```python
from build123d import *

# Parameters (mm, degrees)
F0_W          = 128.129378
F0_H          = 77.922702
F1_DEPTH      = 254
F1_DEPTH_BACK = 25.4
F2_W          = 85.559396
F2_H          = 132.324406
F3_DEPTH      = 254
F4_W          = 107.157492
F4_H          = 126.91684
F5_DEPTH      = 127


with BuildPart() as f1:
    # F0 (on Top) → F1 (new body, two sides)
    with BuildSketch(Plane.XY) as f1_sk:
        Rectangle(F0_W, F0_H)
    extrude(amount=F1_DEPTH)
    extrude(f1_sk.sketch, amount=-F1_DEPTH_BACK)

    # F2 (on Front) → F3 (cut)
    with BuildSketch(Plane.XZ):
        Rectangle(F2_W, F2_H)
    extrude(amount=F3_DEPTH, mode=Mode.SUBTRACT)

    # F4 (on Front) → F5 (cut, symmetric)
    with BuildSketch(Plane.XZ):
        with Locations((0, 155.446574)):
            Rectangle(F4_W, F4_H)
    extrude(amount=F5_DEPTH, both=True, mode=Mode.SUBTRACT)


solid = f1.part
```
Geometry check sheet. Reference: the model listing, model coordinates, mm. A direction names the side the tool comes from. Round coordinates to 2 decimals unless told otherwise and drop trailing zeros. Order: outer loops, then holes, each group sorted by start corner. A loop starts at its lowest first (then second) coordinate and runs counter-clockwise, first axis right, second up. Notation, with made-up numbers: M -14.5,-39 L 15.5,-39 A19 cw 15.5,-11 Z; hole C 7.5,31.25 d3. An arc over 180 degrees is marked long. Answer as CSV lines item,"result".
1) Gauge pin test, flat end, axial feed: pin 1 Ø1.5 at (x, y) = (34.5, -11) entering from -Z. Record the tip position at first contact, or that the pin passes through.
Entries:
pin 1,"z = 66.16"
2) Mould release check, pull along X, two halves, no side actions. Record for faces 1 (the face through (64.065, -1, 116)), 2 (the face through (-64.065, -1, 116)), 3 (the face through (-1, 0, 21)), 4 (the face through (-1, 1, 254)): +X half, -X half, draft (parallel to the pull), parting line (faces both ways), or undercut.
Entries:
face 1,"+X half"
face 2,"-X half"
face 3,"undercut"
face 4,"draft"
3) Thickness scan on probe 1 along X at (y, z) = (-9, 188.5); probe 2 along X at (y, z) = (-16, 41); probe 3 along Z at (x, y) = (-25, -5.5) (3 decimals). Record the ranges inside material, lowest first. Write a range as [from, to].
Entries:
probe 1,"[-64.06, -53.58], [53.58, 64.06]"
probe 2,"[-64.06, -42.78], [42.78, 64.06]"
probe 3,"[66.162, 91.988], [218.905, 254]"
4) Sectioned sample at A-A on z = 155. Record the cut outline in (x, y), and give its area (3 significant figures).
Entries:
outline,"M -64.06,-38.96 L -53.58,-38.96 L -53.58,38.96 L -64.06,38.96 Z; M 53.58,-38.96 L 64.06,-38.96 L 64.06,38.96 L 53.58,38.96 Z"
area,"1,630 mm2"
5) Sectioned sample at C-C on y = 16.5. Record the cut outline in (x, z) (3 decimals).
Entries:
outline,"M -64.065,-25.4 L 64.065,-25.4 L 64.065,254 L -64.065,254 Z; hole M -53.579,91.988 L 53.579,91.988 L 53.579,218.905 L -53.579,218.905 Z"
6) Sectioned sample at D-D on z = 51. Record the cut outline in (x, y).
Entries:
outline,"M -64.06,-38.96 L -42.78,-38.96 L -42.78,0 L 42.78,0 L 42.78,-38.96 L 64.06,-38.96 L 64.06,38.96 L -64.06,38.96 Z"
7) Tool access check on faces 5 (the face through (-1, 9, -25.4)), 6 (the face through (42.78, -19, 20)), 7 (the face through (-1, -1, 218.905)). Record the directions out of +Z, -Z, +X, -X, +Y, -Y that give a thin tool (end or side, any length) a straight path to the whole face; none if there is none.
Entries:
face 5,"-Z, +X, -X, +Y, -Y"
face 6,"-Z, -Y"
face 7,"+Y, -Y"
8) Sectioned sample at B-B on x = -20.5. Record the cut outline in (y, z) (3 decimals), and give its area (3 significant figures).
Entries:
outline,"M -38.961,66.162 L 0,66.162 L 0,-25.4 L 38.961,-25.4 L 38.961,91.988 L -38.961,91.988 Z; M -38.961,218.905 L 38.961,218.905 L 38.961,254 L -38.961,254 Z"
area,"8,310 mm2"
